```python
from build123d import *

# Parameters (mm, degrees)
BOSS_EXTRUDE1_DEPTH = 12.7
BOSS_EXTRUDE3_DEPTH = 12.7
CUT_EXTRUDE1_REACH  = 14.7
CUT_EXTRUDE2_REACH  = 14.7
SKETCH6_W           = 7.112
SKETCH6_H           = 3.302
BOSS_EXTRUDE4_DEPTH = 3.175
SKETCH7_W           = 7.112
SKETCH7_H           = 3.302
BOSS_EXTRUDE5_DEPTH = 3.175


with BuildPart() as part:
    # Sketch1 → Boss-Extrude1 (new body)
    with BuildSketch(Plane(origin=(0, 0, 0), x_dir=(0, 0, -1), z_dir=(1, 0, 0))):
        Polygon((0, 0), (80.01, 0), (80.01, 19.05), (71.12, 19.05), (71.12, 8.89), (8.89, 8.89), (8.89, 19.05), (0, 19.05), align=None)
    extrude(amount=BOSS_EXTRUDE1_DEPTH)

    # Sketch2 → Boss-Extrude3 (add)
    with BuildSketch(Plane.ZY):
        Polygon((-63.5, 12.192), (-70.612, 12.192), (-70.612, 8.89), (-74.93, 8.89), (-74.93, 15.494), (-63.5, 15.494), align=None)
        Polygon((-16.51, 12.192), (-9.398, 12.192), (-9.398, 8.89), (-5.08, 8.89), (-5.08, 15.494), (-16.51, 15.494), align=None)
    extrude(amount=-BOSS_EXTRUDE3_DEPTH)

    # Sketch4 → Cut-Extrude1 (cut, up to next)
    with BuildSketch(Plane.ZY, mode=Mode.PRIVATE) as cut_extrude1_sk1:
        Polygon((-71.12, 15.494), (-75.438, 15.494), (-75.438, 0), (-80.01, 0), (-80.01, 19.05), (-71.12, 19.05), align=None)
    cut_extrude1_tool1 = extrude(cut_extrude1_sk1.sketch, amount=-CUT_EXTRUDE1_REACH, mode=Mode.PRIVATE) & part.part
    add(cut_extrude1_tool1.solids().sort_by_distance((0, 10.686074, -77.05781))[0], mode=Mode.SUBTRACT)

    # Sketch5 → Cut-Extrude2 (cut, up to next)
    with BuildSketch(Plane.ZY, mode=Mode.PRIVATE) as cut_extrude2_sk1:
        Polygon((-8.89, 15.494), (-4.572, 15.494), (-4.572, 0), (0, 0), (0, 19.05), (-8.89, 19.05), align=None)
    cut_extrude2_tool1 = extrude(cut_extrude2_sk1.sketch, amount=-CUT_EXTRUDE2_REACH, mode=Mode.PRIVATE) & part.part
    add(cut_extrude2_tool1.solids().sort_by_distance((0, 10.686074, -2.95219))[0], mode=Mode.SUBTRACT)

    # Sketch6 → Boss-Extrude4 (add)
    with BuildSketch(Plane(origin=(12.7, 0, 0), x_dir=(0, 0, -1), z_dir=(1, 0, 0))):
        with Locations((12.954, 10.541)):
            Rectangle(SKETCH6_W, SKETCH6_H)
    extrude(amount=-BOSS_EXTRUDE4_DEPTH)

    # Sketch7 → Boss-Extrude5 (add)
    with BuildSketch(Plane(origin=(12.7, 0, 0), x_dir=(0, 0, -1), z_dir=(1, 0, 0))):
        with Locations((67.056, 10.541)):
            Rectangle(SKETCH7_W, SKETCH7_H)
    extrude(amount=-BOSS_EXTRUDE5_DEPTH)


solid = part.part
```
The model under review builds one solid part; all positions refer to its coordinate system, in mm. A direction names the side the tool comes from. Give positions to 0.01 mm unless a question says otherwise; leave off trailing zeros. Order: outer loops, then holes, each group sorted by start corner. A loop starts at its lowest first (then second) coordinate and runs counter-clockwise, first axis right, second up. Notation, with made-up numbers: (87.5, 6.25) - (94.5, 6.25) arc R20 cw to (94.5, 28.25) - close; hole circle Ø7 at (32.25, -22.75). An arc over 180 degrees is marked (long way). Use CSV: the item, a comma, the result in double quotes. Start each with the question number.
Q1. We need section B-B, the plane y = 10.75. Write out the cut boundary in (x, z) (3 decimals).
Q2. We need section A-A, the plane z = -10. Write out the cut boundary in (x, y) (3 decimals), and give its area (3 significant figures).
Q3. Clearance check with flat-ended pins moving along their axes: pin 1 Ø5 at (y, z) = (12.5, -39.5) entering from -X (1 decimal); pin 2 Ø1.7 at (y, z) = (10, -68.5) entering from -X (3 decimals); pin 3 Ø4 at (x, z) = (2, -27.5) entering from +Y. State where each tip first meets the part, or that it passes through.
Q4. We need section D-D, the plane x = 7.25. Write out the cut boundary in (y, z).
Q5. To check wall thickness, follow line 1 along Z through (x, y) = (5, 14.25); line 2 along Y through (x, z) = (6.25, -51.5); line 3 along Z through (x, y) = (4, 9.5). State the ranges of each line that lie inside material, in increasing order. Write a range as [from, to].
Q6. The part is to be moulded in two halves that separate along Y. For faces 4 (the flat face through (6, 15.494, -70)), 5 (the flat face through (8, 14, -16.51)), 6 (the flat face through (9.525, 11, -13)), say which applies: +Y half, -Y half, draft (parallel to the pull), parting line (faces both ways), or undercut.
Q7. Tool access review of faces 1 (the flat face through (12.7, 6, -40)), 2 (the flat face through (8, 14, -63.5)), 3 (the flat face through (5, 11, -9.398)): name each direction out of +Z, -Z, +X, -X, +Y, -Y from which nothing blocks a thin tool from reaching the whole face with its end or side.
Q8. We need section C-C, the plane x = 11.5. Write out the cut boundary in (y, z), and give its area (3 significant figures).
Outcome:
1,outline,"(0, -75.438) - (12.7, -75.438) - (12.7, -63.5) - (9.525, -63.5) - (9.525, -70.612) - (0, -70.612) - close; (0, -9.398) - (9.525, -9.398) - (9.525, -16.51) - (12.7, -16.51) - (12.7, -4.572) - (0, -4.572) - close"
2,outline,"(0, 0) - (12.7, 0) - (12.7, 15.494) - (0, 15.494) - (0, 12.192) - (9.525, 12.192) - (9.525, 8.89) - (0, 8.89) - close"
2,area,"165 mm^2"
3,pin 1,"passes through"
3,pin 2,"stops at x = 9.525"
3,pin 3,"stops at y = 8.89"
4,outline,"(0, -75.44) - (15.49, -75.44) - (15.49, -63.5) - (12.19, -63.5) - (12.19, -70.61) - (8.89, -70.61) - (8.89, -9.4) - (12.19, -9.4) - (12.19, -16.51) - (15.49, -16.51) - (15.49, -4.57) - (0, -4.57) - close"
5,line 1,"z = [-75.44, -63.5], [-16.51, -4.57]"
5,line 2,"y = [0, 8.89]"
5,line 3,"z = [-75.44, -70.61], [-9.4, -4.57]"
6,face 4,"+Y half"
6,face 5,"draft"
6,face 6,"undercut"
7,face 1,"+Z, -Z, +X, +Y, -Y"
7,face 2,"+X, -X, +Y"
7,face 3,"-X"
8,outline,"(0, -75.44) - (15.49, -75.44) - (15.49, -63.5) - (8.89, -63.5) - (8.89, -16.51) - (15.49, -16.51) - (15.49, -4.57) - (0, -4.57) - close"
8,area,"788 mm^2"
